```python
from build123d import *

# Parameters (mm, degrees)
F0_W      = 15.8
F0_H      = 7.83
F1_DEPTH  = 3.3
F3_DEPTH  = 9.37
F4_R      = 1.46
F5_DEPTH  = 3.31
F6_W      = 12.78
F6_H      = 4.59
F7_DEPTH  = 25
F8_W      = 15.7957389019
F8_H      = 7.7149206772
F9_DEPTH  = 2
F10_R     = 1.57
F10_R_2   = 0.72
F11_DEPTH = 3


with BuildPart() as f1:
    # F0 (on Top) → F1 (new body)
    with BuildSketch(Plane.XY):
        with Locations((-0.7034245188, -3.915)):
            Rectangle(F0_W, F0_H)
    extrude(amount=-F1_DEPTH)

    # F2 (on Top) → F3 (join)
    with BuildSketch(Plane.XY):
        with BuildLine():
            Line((3.4065754812, 0), (-4.2734245188, 0))
            Line((-4.2734245188, 0), (-4.2734245188, -1.65))
            Line((-4.2734245188, -1.65), (-1.3598001921, -1.65))
            ThreePointArc((-1.3598001921, -1.65), (-0.4334245188, -0.7236243267), (0.4929511545, -1.65))
            Line((0.4929511545, -1.65), (3.4065754812, -1.65))
            Line((3.4065754812, -1.65), (3.4065754812, 0))
        make_face()
        with BuildLine():
            ThreePointArc((0.4929511545, -1.65), (-0.4334245188, -0.7236243267), (-1.3598001921, -1.65))
            Line((-1.3598001921, -1.65), (0.4929511545, -1.65))
        make_face()
        with BuildLine():
            Line((0.4929511545, -1.65), (-1.3598001921, -1.65))
            ThreePointArc((-1.3598001921, -1.65), (-0.4334245188, -2.5763756733), (0.4929511545, -1.65))
        make_face()
    extrude(amount=F3_DEPTH)

    # F4 (on Front) → F5 (join)
    with BuildSketch(Plane.XZ):
        with Locations((-0.2993772502, 7.8826601838)):
            Circle(F4_R)
    extrude(amount=F5_DEPTH)

    # F6 (on Top) → F7 (cut)
    with BuildSketch(Plane.XY):
        with Locations((-0.7034245188, -3.915)):
            Rectangle(F6_W, F6_H)
    extrude(amount=-F7_DEPTH, mode=Mode.SUBTRACT)

    # F8 (on Top) → F9 (join)
    with BuildSketch(Plane.XY):
        with Locations((-0.7554732729, -3.8574603386)):
            Rectangle(F8_W, F8_H)
    extrude(amount=-F9_DEPTH)

    # F10 (on Top) → F11 (join)
    with BuildSketch(Plane.XY):
        with Locations((-0.4749980129, -3.7706719508)):
            Circle(F10_R)
        with Locations((-0.4749980129, -3.7706719508)):
            Circle(F10_R_2, mode=Mode.SUBTRACT)
    extrude(amount=-F11_DEPTH)


solid = f1.part
```
Geometry: final body of the model. Coordinates: model frame, mm. A direction names the side the tool comes from. Give positions to 0.01 mm unless a question says otherwise; leave off trailing zeros. Order: outer loops, then holes, each group sorted by start corner. A loop starts at its lowest first (then second) coordinate and runs counter-clockwise, first axis right, second up. Notation, with made-up numbers: M 15,-15.75 L 39,-15.75 A17 cw 39,13.25 Z; hole C 41.5,52.5 d1. An arc over 180 degrees is marked long. Answer as CSV lines item,"result". Start each with the question number.
1) Line query: line 1 (Y direction, x = 3, z = -2.5); line 2 (Z direction, x = -3.5, y = -3.25); line 3 (X direction, y = -0.25, z = 5.5). Output: solid intervals per line, ascending. Write a range as from..to.
2) First-contact query: P1, Ø6, axis at x = -5, z = 3.5, coming from the -Y side; P2, Ø0.8, axis at y = -0.5, z = 4.5, coming from the +X side; P3, Ø1.5, axis at x = -1, z = 7.5, coming from the -Y side; P4, Ø1.5, axis at y = -4.5, z = 4.5, coming from the +X side. Flat tips, straight axial feed; report the tip coordinate or a pass-through.
3) Cut plane C-C (z = 0.5). Output: boundary loops of the cut face in (x, y).
4) Cut plane A-A (z = -2.5). Output: boundary loops of the cut face in (x, y) (3 decimals), then the cut area to 3 significant figures.
5) Cut plane D-D (x = -7.5). Output: boundary loops of the cut face in (y, z).
6) Mould query, pull axis X, two halves, no side actions, for faces 4 (the flat face through (-1, -4, 0)), 5 (the flat face through (7.197, -4, -2)), 6 (the flat face through (-2.2, -3.9, -2)), 7 (the cylindrical face through (-0.454, -2.576, 3.391)). Classes: +X half, -X half, draft (parallel to the pull), parting line (faces both ways), or undercut.
7) Cut plane B-B (y = -0.5). Output: boundary loops of the cut face in (x, z), then the cut area to 3 significant figures.
8) Set-up query: faces 1 (the flat face through (-1, -6.21, -3)), 2 (the flat face through (2, -1.65, 5)), 3 (the flat face through (3.407, -1, 5)). Return all of +Z, -Z, +X, -X, +Y, -Y with unobstructed straight access to the full face (end or side cutting, diameter ignored); none if empty.
Findings below:
1,line 1,"y = -7.83..-6.21, -1.62..0"
1,line 2,"z = -2..0"
1,line 3,"x = -4.27..3.41"
2,P1,"stops at y = -1.65"
2,P2,"stops at x = 3.41"
2,P3,"stops at y = -3.31"
2,P4,"passes through"
3,outline,"M -4.27,-1.65 L -1.36,-1.65 A0.93 ccw 0.49,-1.65 L 3.41,-1.65 L 3.41,0 L -4.27,0 Z"
4,outline,"M -8.603,-7.83 L 7.197,-7.83 L 7.197,0 L -8.603,0 Z; C -0.475,-3.771 d3.14; hole M -7.093,-6.21 L 5.687,-6.21 L 5.687,-1.62 L -7.093,-1.62 Z; hole C -0.475,-3.771 d1.44"
4,area,"71.2 mm²"
5,outline,"M -7.83,-3.3 L 0,-3.3 L 0,0 L -7.83,0 Z"
6,face 4,"draft"
6,face 5,"+X half"
6,face 6,"undercut"
6,face 7,"parting line"
7,outline,"M -8.65,-2 L -8.6,-2 L -8.6,-3.3 L 7.2,-3.3 L 7.2,0 L 3.41,0 L 3.41,9.37 L -4.27,9.37 L -4.27,0 L -8.65,0 Z"
7,area,"124 mm²"
8,face 1,"-Z"
8,face 2,"+X, -Y"
8,face 3,"+Z, +X, +Y, -Y"
